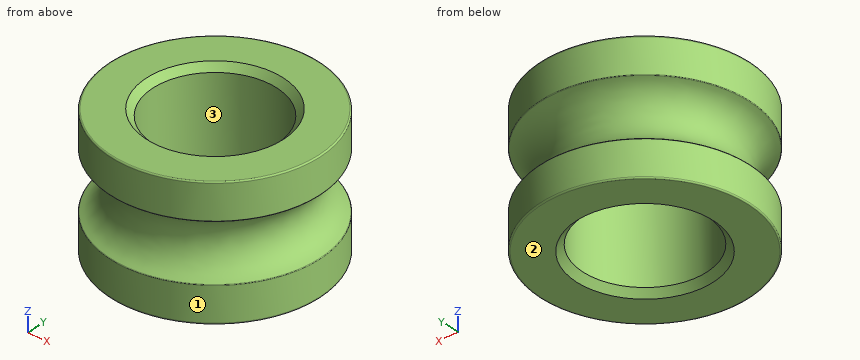
```python
from build123d import *


with BuildPart() as part:
    # Inner Bearing Race Profile → Inner Bearing Race (revolve)
    with BuildSketch(Plane(origin=(0, 0, 0), x_dir=(0, 0, -1), z_dir=(1, 0, 0)), mode=Mode.PRIVATE) as inner_bearing_race_sk:
        with BuildLine():
            Line((2.24028, 2.38125), (2.4892, 2.63017))
            Line((2.4892, 2.63017), (2.4892, 3.975414011))
            ThreePointArc((2.4892, 3.975414011), (2.474321024, 4.011335035), (2.4384, 4.026214011))
            Line((2.4384, 4.026214011), (1.12493032, 4.026214011))
            ThreePointArc((1.12493032, 4.026214011), (1.109994783, 4.021358833), (1.100769063, 4.008649422))
            ThreePointArc((1.100769063, 4.008649422), (0, 3.208419705), (-1.100769063, 4.008649422))
            ThreePointArc((-1.100769063, 4.008649422), (-1.109994783, 4.021358833), (-1.12493032, 4.026214011))
            Line((-1.12493032, 4.026214011), (-2.4384, 4.026214011))
            ThreePointArc((-2.4384, 4.026214011), (-2.474321024, 4.011335035), (-2.4892, 3.975414011))
            Line((-2.4892, 3.975414011), (-2.4892, 2.63017))
            Line((-2.4892, 2.63017), (-2.24028, 2.38125))
            Line((-2.24028, 2.38125), (2.24028, 2.38125))
        make_face()
    revolve(inner_bearing_race_sk.sketch.rotate(Axis((0, 0, 2.4892), (0, 0, -1)), 90), axis=Axis((0, 0, 2.4892), (0, 0, -1)))


solid = part.part
```
CAD build for the part. Positions are in the model's coordinates, mm. Face numbers are marked on the shaded views. Give positions to 0.01 mm unless a question says otherwise; leave off trailing zeros. Write each loop counter-clockwise with the first axis right and the second up, starting at its lowest first coordinate (ties: lowest second). Pieces come first, ordered by that corner, then holes. Notation, with made-up numbers: (13.25, 12.25) -> (71.25, 12.25) arc R21 ccw to (71.25, 34.25) -> close; hole circle Ø7 at (64.25, 58.25). An arc over 180 degrees is marked (long way). Write each question's results on one line, items separated by ' | '.
1. Two-plate mould, pull along X, no slides. Class the marked faces 1, 2 and 3: pulls with the +X half, pulls with the -X half, needs draft (parallel to the pull), parting line crosses it, or undercut.
Geometry check:
face 1: parting line crosses it | face 2: needs draft | face 3: undercut
2. Wall check: probe 1 along Y at (x, z) = (0, -1.9); probe 2 along Y at (x, z) = (-1.25, -0.7); probe 3 along X at (y, z) = (-1, -2). Give the ranges that are in metal, low to high. Write a range as [from, to].
Geometry check:
probe 1: [-4.03, -2.38], [2.38, 4.03] | probe 2: [-3.21, -2.03], [2.03, 3.21] | probe 3: [-3.9, -2.16], [2.16, 3.9]
3. Cut at C-C, the plane z = -1.95. Write the cut outline in (x, y).
Geometry check:
outline: circle Ø8.05 at (0, 0); hole circle Ø4.76 at (0, 0)
4. Cut at D-D, the plane z = 0.3. Write the cut outline in (x, y), then the cut area to 3 significant figures.
Geometry check:
outline: circle Ø6.5 at (0, 0); hole circle Ø4.76 at (0, 0) | area: 15.3 mm²
5. Drop flat-ended pins along their axis: P1, Ø1.5, axis at y = 2, z = -1, coming from the -X side; P2, Ø1, axis at y = 0, z = 0, coming from the +X side. Give the stop position or say it passes through.
Geometry check:
P1: x = -3.82 | P2: x = 3.32
